For this review, use the dimensioned drawing (mm, ordinates from the lowest corner) and the shaded views. Give positions to 0.01 mm unless a question says otherwise; leave off trailing zeros. Order: outer loops, then holes, each group sorted by start corner. A loop starts at its lowest first (then second) coordinate and runs counter-clockwise, first axis right, second up.
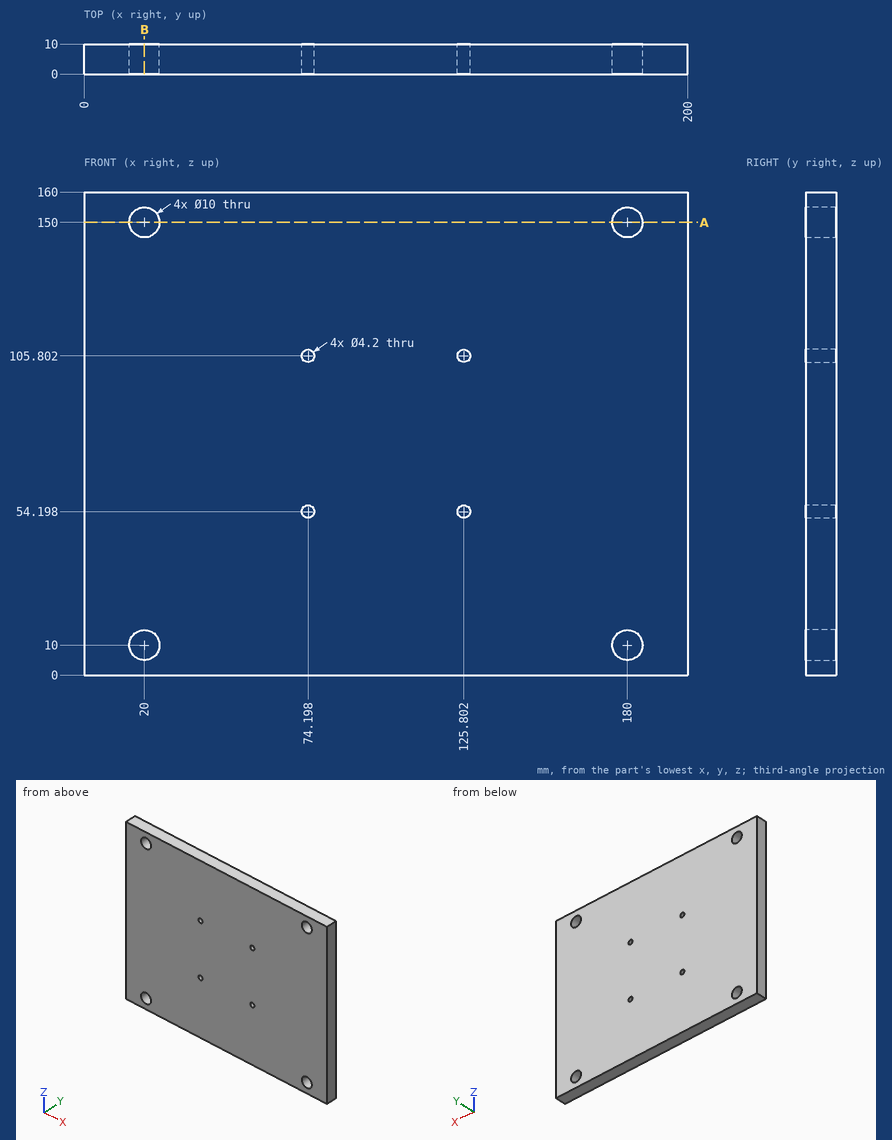
1. To check wall thickness, follow line 1 (Z direction, x = 180, y = 6.5); line 2 (X direction, y = 7, z = 10); line 3 (X direction, y = 1, z = 13). State the ranges of each line that lie inside material, in increasing order.
2. Take a section at A-A (z = 150). Write out the cut boundary in (x, y).
3. Take a section at B-B (x = 20). Write out the cut boundary in (y, z), and give its area (3 significant figures).
Answer:
1. line 1: z = 0 to 5, 15 to 145, 155 to 160
1. line 2: x = 0 to 15, 25 to 175, 185 to 200
1. line 3: x = 0 to 16, 24 to 176, 184 to 200
2. outline: (0, 0) - (15, 0) - (15, 10) - (0, 10) - close; (25, 0) - (175, 0) - (175, 10) - (25, 10) - close; (185, 0) - (200, 0) - (200, 10) - (185, 10) - close
3. outline: (0, 0) - (10, 0) - (10, 5) - (0, 5) - close; (0, 15) - (10, 15) - (10, 145) - (0, 145) - close; (0, 155) - (10, 155) - (10, 160) - (0, 160) - close
3. area: 1,400 mm2
